```python
from build123d import *

# Parameters (mm, degrees)
PAD_DEPTH = 2


with BuildPart() as part:
    # Sketch → Pad (new body)
    with BuildSketch(Plane.XZ):
        Polygon((0, 1.5), (8, 1.5), (8, -1.5), (0, -1.5), (-5, 0), align=None)
    extrude(amount=PAD_DEPTH)


solid = part.part
```
Geometry: final body of the model. Coordinates: model frame, mm. Coordinates: 2 decimals unless noted, no trailing zeros. Order: outer loops, then holes, each group sorted by start corner. A loop starts at its lowest first (then second) coordinate and runs counter-clockwise, first axis right, second up. Notation, with made-up numbers: (-31, -19.75) - (-24, -19.75) arc R17 cw to (-24, 2.25) - close; hole circle Ø10 at (34.5, 18). An arc over 180 degrees is marked (long way). Write each question's results on one line, items separated by ' | '.
1) Section C-C, the plane x = -2.5. Return loops of the section in (y, z), plus the area to 3 significant figures.
Results list:
outline: (-2, -0.75) - (0, -0.75) - (0, 0.75) - (-2, 0.75) - close | area: 3.00 mm^2
2) Line query: line 1 (Z direction, x = -0.5, y = -0.25); line 2 (Z direction, x = -1.75, y = -0.6) (3 decimals). Output: solid intervals per line, ascending. Write a range as from..to.
Results list:
line 1: -1.35..1.35 | line 2: -0.975..0.975
3) Section A-A, the plane y = -0.45. Return loops of the section in (x, z), plus the area to 3 significant figures.
Results list:
outline: (-5, 0) - (0, -1.5) - (8, -1.5) - (8, 1.5) - (0, 1.5) - close | area: 31.5 mm^2
4) Section B-B, the plane z = -0.6. Return loops of the section in (x, y), plus the area to 3 significant figures.
Results list:
outline: (-3, -2) - (8, -2) - (8, 0) - (-3, 0) - close | area: 22.0 mm^2
